from build123d import *

# Parameters (mm, degrees)
F1_DEPTH = 40
F3_D     = 4
F4_W     = 9
F4_H     = 1.5
F5_DEPTH = 1.75
F6_W     = 9
F6_H     = 1.5
F7_DEPTH = 1.75
F8_W     = 10.8425548855
F8_H     = 10.4324881697
F8_W_2   = 3.9074451145
F8_H_2   = 6.5675118303
F9_DEPTH = 9.001


with BuildPart() as f1:
    # F0 (on Front) → F1 (new body)
    with BuildSketch(Plane.XZ):
        Polygon((0, 9), (0, 0), (35.5, 0), (35.5, 1.5), align=None)
    extrude(amount=F1_DEPTH)

    # F3 (through all)
    with Locations(Plane(origin=(0, 0, 0), x_dir=(1, 0, 0), z_dir=(0, 0, -1))):
        with Locations((3.75, 34), (31.75, 34), (31.75, 6), (3.75, 6)):
            Hole(F3_D / 2)

    # F4 (on face) → F5 (join)
    with BuildSketch(Plane(origin=(0, 0, 0), x_dir=(0, -1, 0), z_dir=(-1, 0, 0))):
        with Locations((29.5, 0.75)):
            Rectangle(F4_W, F4_H)
        with Locations((10.5, 0.75)):
            Rectangle(F4_W, F4_H)
    extrude(amount=F5_DEPTH)

    # F6 (on face) → F7 (join)
    with BuildSketch(Plane.YZ.offset(35.5)):
        with Locations((-10.5, 0.75)):
            Rectangle(F6_W, F6_H)
        with Locations((-29.5, 0.75)):
            Rectangle(F6_W, F6_H)
    extrude(amount=F7_DEPTH)

    # F8 (on face) → F9 (cut, through all)
    with BuildSketch(Plane(origin=(0, 0, 0), x_dir=(1, 0, 0), z_dir=(0, 0, -1))):
        with Locations((23.1712774428, 25.2162440849)):
            Rectangle(F8_W, F8_H)
        with Locations((12.3287225572, 14.7837559151)):
            Rectangle(F8_W, F8_H)
        with Locations((12.3287225572, 25.2162440849)):
            Rectangle(F8_W, F8_H)
        with Locations((23.1712774428, 14.7837559151)):
            Rectangle(F8_W, F8_H)
        with Locations((30.5462774428, 25.2162440849)):
            Rectangle(F8_W_2, F8_H)
        with Locations((30.5462774428, 14.7837559151)):
            Rectangle(F8_W_2, F8_H)
        with Locations((4.9537225572, 14.7837559151)):
            Rectangle(F8_W_2, F8_H)
        with Locations((4.9537225572, 25.2162440849)):
            Rectangle(F8_W_2, F8_H)
        with Locations((12.3287225572, 33.7162440849)):
            Rectangle(F8_W, F8_H_2)
        with Locations((23.1712774428, 33.7162440849)):
            Rectangle(F8_W, F8_H_2)
        with Locations((23.1712774428, 6.2837559151)):
            Rectangle(F8_W, F8_H_2)
        with Locations((12.3287225572, 6.2837559151)):
            Rectangle(F8_W, F8_H_2)
    extrude(amount=-F9_DEPTH, mode=Mode.SUBTRACT)


solid = f1.part
Could you check a few things on this model? Use its own coordinates, in mm. A direction names the side the tool comes from. Round coordinates to 2 decimals unless told otherwise and drop trailing zeros. Write each loop counter-clockwise with the first axis right and the second up, starting at its lowest first coordinate (ties: lowest second). Pieces come first, ordered by that corner, then holes. Notation, with made-up numbers: (6, 18.5) - (65, 18.5) arc R7 ccw to (65, 24.5) - close; hole circle Ø4 at (-30, 48.5). An arc over 180 degrees is marked (long way). Put each result on its own line as item: value. Start each with the question number.
(1) I want a section at D-D, the plane x = 3.75. Please give me the cut outline in (y, z).
(2) Thinking about a two-plate mould opening in Y: for faces 1 (the flat face through (-1, -25, 1)), 2 (the flat face through (33.776, -19.72, 1.864)), 3 (the flat face through (14, 0, 4)), which applies, released by +Y, released by -Y, zero draft, split by the parting line, or undercut?
(3) I want a section at A-A, the plane y = -15.5. Please give me the cut outline in (x, z).
(4) I want a section at B-B, the plane z = 3.75. Please give me the cut outline in (x, y).
(5) Will these pins go through, and if not, where does the flat tip stop? pin 1 (1.7 mm diameter, centred on y = -23.5, z = 1, fed in from -X); pin 2 (1.2 mm diameter, centred on y = -2, z = 0.5, fed in from +X); pin 3 (0.5 mm diameter, centred on x = 36, y = -27.5, fed in from +Z).
(6) I need wall thicknesses on probe 1 along X at (y, z) = (-34, 2); probe 2 along Y at (x, z) = (31.75, 1.8); probe 3 along X at (y, z) = (-34, 5.5). Which ranges of each line are inside material? Lowest first, please.
(7) I want a section at C-C, the plane x = 33. Please give me the cut outline in (y, z).
(8) For faces 4 (the flat face through (36, -34, 1)), 5 (the flat face through (36, -15, 1)), 6 (the flat face through (3, -20, 4)), 7 (the flat face through (-1, -29, 1.5)), which set-ups out of +Z, -Z, +X, -X, +Y, -Y let a thin tool reach every point of the face, with its end or its side?
Here are the results:
1. outline: (-40, 0) - (-36, 0) - (-36, 8.21) - (-40, 8.21) - close; (-32, 0) - (-30.43, 0) - (-30.43, 8.21) - (-32, 8.21) - close; (-9.57, 0) - (-8, 0) - (-8, 8.21) - (-9.57, 8.21) - close; (-4, 0) - (0, 0) - (0, 8.21) - (-4, 8.21) - close
2. face 1: undercut
2. face 2: zero draft
2. face 3: released by +Y
3. outline: (0, 0) - (3, 0) - (3, 8.37) - (0, 9) - close; (32.5, 0) - (35.5, 0) - (35.5, 1.5) - (32.5, 2.13) - close
4. outline: (0, -40) - (24.85, -40) - (24.85, -37) - (6.91, -37) - (6.91, -30.43) - (3, -30.43) - (3, -9.57) - (6.91, -9.57) - (6.91, -3) - (24.85, -3) - (24.85, 0) - (0, 0) - close; hole circle Ø4 at (3.75, -34); hole circle Ø4 at (3.75, -6)
5. pin 1: stops at x = 0
5. pin 2: stops at x = 35.5
5. pin 3: stops at z = 1.5
6. probe 1: x = 0 to 1.75, 5.75 to 6.91, 28.59 to 29.75
6. probe 2: y = -40 to -36, -32 to -30.43, -9.57 to -8, -4 to 0
6. probe 3: x = 0 to 1.75, 5.75 to 6.91
7. outline: (-40, 0) - (-35.56, 0) - (-35.56, 2.03) - (-40, 2.03) - close; (-32.44, 0) - (-7.56, 0) - (-7.56, 2.03) - (-32.44, 2.03) - close; (-4.44, 0) - (0, 0) - (0, 2.03) - (-4.44, 2.03) - close
8. face 4: +Z, -Z, +X, -Y
8. face 5: +Z, -Z, +X
8. face 6: +Z, -Z
8. face 7: +Z, -X, +Y, -Y
